from build123d import *

# Parameters (mm, degrees)
F0_R     = 3
F1_DEPTH = 8
F3_DEPTH = 3
F4_R     = 2
F5_DEPTH = 25
F6_SIZE  = 0.99999


# Not quite as in the source:
# - a fillet or chamfer is up to 0.001 mm smaller than in the source, because OpenCascade refuses the exact size


with BuildPart() as f1:
    # F0 (on Front) → F1 (new body)
    with BuildSketch(Plane.XZ):
        Circle(F0_R)
    extrude(amount=F1_DEPTH)

    # F2 (on face) → F3 (cut)
    with BuildSketch(Plane.XZ.offset(8)):
        Polygon((2, 1.1547005384), (0, 2.3094010768), (-2, 1.1547005384), (-2, -1.1547005384), (0, -2.3094010768), (2, -1.1547005384), align=None)
    extrude(amount=-F3_DEPTH, mode=Mode.SUBTRACT)

    # F4 (on face) → F5 (cut)
    with BuildSketch(Plane.XZ.offset(5)):
        Circle(F4_R)
    extrude(amount=-F5_DEPTH, mode=Mode.SUBTRACT)

    # F6 (size 1 in the source; OpenCascade refuses exactly that, so slightly less here)
    f6_edges = [f1.edges().sort_by_distance(p)[0] for p in [
        (-3, 0, 0),
    ]]
    chamfer(f6_edges, length=F6_SIZE)


solid = f1.part
Geometry check sheet. Reference: the model listing, model coordinates, mm. A direction names the side the tool comes from. Give positions to 0.01 mm unless a question says otherwise; leave off trailing zeros. Order: outer loops, then holes, each group sorted by start corner. A loop starts at its lowest first (then second) coordinate and runs counter-clockwise, first axis right, second up.
1. Depth check by flat-ended pin: pin 1 (2.5 mm diameter, centred on x = 0, z = 0, fed in from -Y). Enter the tip coordinate at first touch or a pass-through.
Completed:
pin 1: passes through
2. Scan lines: line 1 (Z direction, x = 0, y = -3.85); line 2 (X direction, y = -2.25, z = 1.15). Record each from-to range of solid material in increasing order.
Completed:
line 1: z = -3 to -2, 2 to 3
line 2: x = -2.77 to -1.64, 1.64 to 2.77
3. Sectioned sample at A-A (y = -3). Record the boundary of the cut face in (x, z), then the cut area to 3 significant figures.
Completed:
outline: circle Ø6 at (0, 0); hole circle Ø4 at (0, 0)
area: 15.7 mm2
4. Access from +Z, -Z, +X, -X, +Y, -Y to the whole of each face (thin tool, end or side, straight path). Record for faces 1 (the face through (-2, -7, 0)), 2 (the face through (-3, -4, 0)).
Completed:
face 1: -Y
face 2: +Y, -Y
